Input: part model. Units: mm. Frame: model coordinates. Face numbers are marked on the shaded views. A direction names the side the tool comes from. Give positions to 0.01 mm unless a question says otherwise; leave off trailing zeros. Loops run counter-clockwise (first coordinate to the right, second up) from the corner with the lowest first, then second, coordinate; pieces in that order, holes last. Notation, with made-up numbers: (65, 34.5) - (78, 34.5) arc R30 cw to (78, 67.5) - close; hole circle Ø3 at (24, 71.25). An arc over 180 degrees is marked (long way). Answer as a JSON object with one key per item and string values.
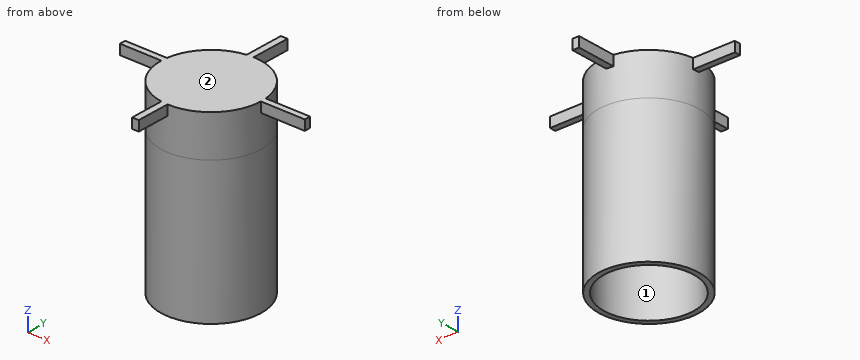
from build123d import *

# Parameters (mm, degrees)
F0_W     = 3.9692334831
F0_H     = 103.9218027145
F2_DEPTH = 31.75
F3_W     = 64.669739455
F3_H     = 4.6622371301
F3_W_2   = 5.0883553922
F3_H_2   = 63.7673670426
F3_W_3   = 72.5153312087
F3_H_3   = 63.9177635312
F4_DEPTH = 7.62


with BuildPart() as f1:
    # F0 (on Front) → F1 (revolve)
    with BuildSketch(Plane.XZ):
        Polygon((10.5738220736, 29.8581575043), (-27.7522327378, 29.8581575043), (-27.7522327378, 25.5280886777), (6.6045885906, 25.5280886777), (10.5738220736, 25.5280886777), align=None)
        with Locations((8.5892053321, -26.4328126796)):
            Rectangle(F0_W, F0_H)
    revolve(axis=Axis((-27.7522327378, 0, 22.6518814452), (0, 0, 1)))

    # F2 (add): a face of the model
    f2_faces = [f1.faces().sort_by_distance(p)[0] for p in [
        (-27.7522327378, 0, 29.8581575043),
    ]]
    extrude(f2_faces, amount=F2_DEPTH)

    # F3 (on face) → F4 (join)
    with BuildSketch(Plane.XY.offset(61.6081575043)):
        with Locations((-65.5721072108, 2.3311185651)):
            Rectangle(F3_W, F3_H)
        with Locations((-30.6930597872, 36.5459206514)):
            Rectangle(F3_W_2, F3_H_2)
        with Locations((-30.6930597872, 2.3311185651)):
            Rectangle(F3_W_2, F3_H)
        with Locations((8.1087835133, 2.3311185651)):
            Rectangle(F3_W_3, F3_H)
        with Locations((-30.6930597872, -31.9588817656)):
            Rectangle(F3_W_2, F3_H_3)
    extrude(amount=-F4_DEPTH)


solid = f1.part
Item 1: Material intervals for line 1 (Z direction, x = -5, y = -18); line 2 (Y direction, x = 0.5, z = 4.5); line 3 (X direction, y = -29.5, z = -8.5), sorted ascending. Write a range as [from, to].
Geometry check:
{"line 1": "z = [25.53, 61.61]", "line 2": "y = [-25.9, -19.55], [19.55, 25.9]", "line 3": "x = [-52.22, -45.36], [-10.14, -3.29]"}
Item 2: Cut plane B-B (x = -52). Return loops of the section in (y, z), then the cut area to 3 significant figures.
Geometry check:
{"outline": "(-29.68, -78.39) - (-24.34, -78.39) - (-24.34, 25.53) - (24.34, 25.53) - (24.34, -78.39) - (29.68, -78.39) - (29.68, 61.61) - (-29.68, 61.61) - close", "area": "3,250 mm2"}
Item 3: Cut plane C-C (z = -2.5). Return loops of the section in (x, y).
Geometry check:
{"outline": "circle Ø76.65 at (-27.75, 0); hole circle Ø68.71 at (-27.75, 0)"}
Item 4: Contact query for flat-ended pins moving along their axis: P1, Ø20.5, axis at x = -23.5, y = -0.5, coming from the -Z side; P2, Ø4, axis at x = 24, z = 58, coming from the -Y side; P3, Ø6, axis at x = -79, z = 59, coming from the +Y side. Output: stop coordinate, or through.
Geometry check:
{"P1": "stops at z = 25.53", "P2": "stops at y = 0", "P3": "stops at y = 4.66"}
Item 5: Cut plane D-D (z = 41). Return loops of the section in (x, y), then the cut area to 3 significant figures.
Geometry check:
{"outline": "circle Ø76.65 at (-27.75, 0)", "area": "4,610 mm2"}
Item 6: Access query for the marked faces 1 and 2. Directions: +Z, -Z, +X, -X, +Y, -Y. A direction counts if a zero-diameter tool reaches every point of the face in a straight line with its end or side. Return the directions, or none.
Geometry check:
{"face 1": "-Z", "face 2": "+Z, +X, -X, +Y, -Y"}
Item 7: Cut plane A-A (y = -11.5). Return loops of the section in (x, z).
Geometry check:
{"outline": "(-64.31, -78.39) - (-60.13, -78.39) - (-60.13, 25.53) - (4.62, 25.53) - (4.62, -78.39) - (8.81, -78.39) - (8.81, 61.61) - (-64.31, 61.61) - close"}
